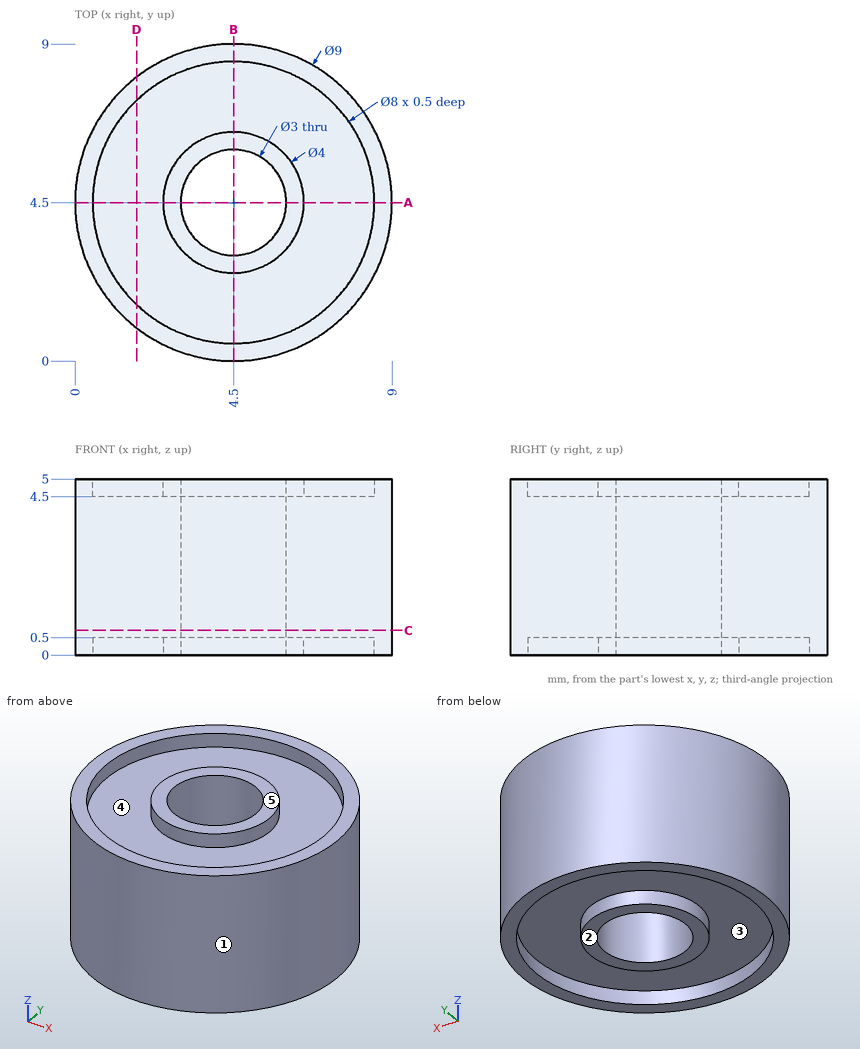
Design review of the part shown in the three views and the two pictorial views. Dimensions are in mm from the part's minimum x, y and z. A direction names the side the tool comes from. Give positions to 0.01 mm unless a question says otherwise; leave off trailing zeros. Write each loop counter-clockwise with the first axis right and the second up, starting at its lowest first coordinate (ties: lowest second). Pieces come first, ordered by that corner, then holes.
(1) Mouldability with a two-part tool opening along X and no side actions: class the marked faces 1, 2 and 3 as +X half, -X half, draft (parallel to the pull), parting line (faces both ways), or undercut.
Checked values:
face 1: parting line
face 2: draft
face 3: undercut
(2) Add section A-A (y = 4.5). Give the boundary of the cut face in (x, z).
Checked values:
outline: (0, 0) - (0.5, 0) - (0.5, 0.5) - (2.5, 0.5) - (2.5, 0) - (3, 0) - (3, 5) - (2.5, 5) - (2.5, 4.5) - (0.5, 4.5) - (0.5, 5) - (0, 5) - close; (6, 0) - (6.5, 0) - (6.5, 0.5) - (8.5, 0.5) - (8.5, 0) - (9, 0) - (9, 5) - (8.5, 5) - (8.5, 4.5) - (6.5, 4.5) - (6.5, 5) - (6, 5) - close
(3) Clearance check with flat-ended pins moving along their axes: pin 1 Ø1.5 at (x, y) = (7, 3) entering from -Z; pin 2 Ø3 at (y, z) = (7, 3.5) entering from -X; pin 3 Ø1.5 at (y, z) = (7.5, 1.5) entering from +X; pin 4 Ø1.5 at (x, y) = (6, 7.5) entering from +Z. State where each tip first meets the part, or that it passes through.
Checked values:
pin 1: stops at z = 0.5
pin 2: stops at x = 0.11
pin 3: stops at x = 8.4
pin 4: stops at z = 5
(4) Wall thickness on line 1 along Y through (x, z) = (4.5, 0.2); line 2 along Z through (x, y) = (3.5, 0.75); line 3 along X through (y, z) = (5.5, 4.35): over which ranges is each line inside the solid? List them lowest first.
Checked values:
line 1: y = 0 to 0.5, 2.5 to 3, 6 to 6.5, 8.5 to 9
line 2: z = 0.5 to 4.5
line 3: x = 0.11 to 3.38, 5.62 to 8.89
(5) Add section C-C (z = 0.7). Give the boundary of the cut face in (x, y).
Checked values:
outline: circle Ø9 at (4.5, 4.5); hole circle Ø3 at (4.5, 4.5)
(6) Tool access review of the marked faces 4 and 5: name each direction out of +Z, -Z, +X, -X, +Y, -Y from which nothing blocks a thin tool from reaching the whole face with its end or side.
Checked values:
face 4: +Z
face 5: +Z, +X, -X, +Y, -Y
(7) Add section D-D (x = 1.75). Give the boundary of the cut face in (y, z), and give its area (3 significant figures).
Checked values:
outline: (0.94, 0) - (1.6, 0) - (1.6, 0.5) - (7.4, 0.5) - (7.4, 0) - (8.06, 0) - (8.06, 5) - (7.4, 5) - (7.4, 4.5) - (1.6, 4.5) - (1.6, 5) - (0.94, 5) - close
area: 29.8 mm2
